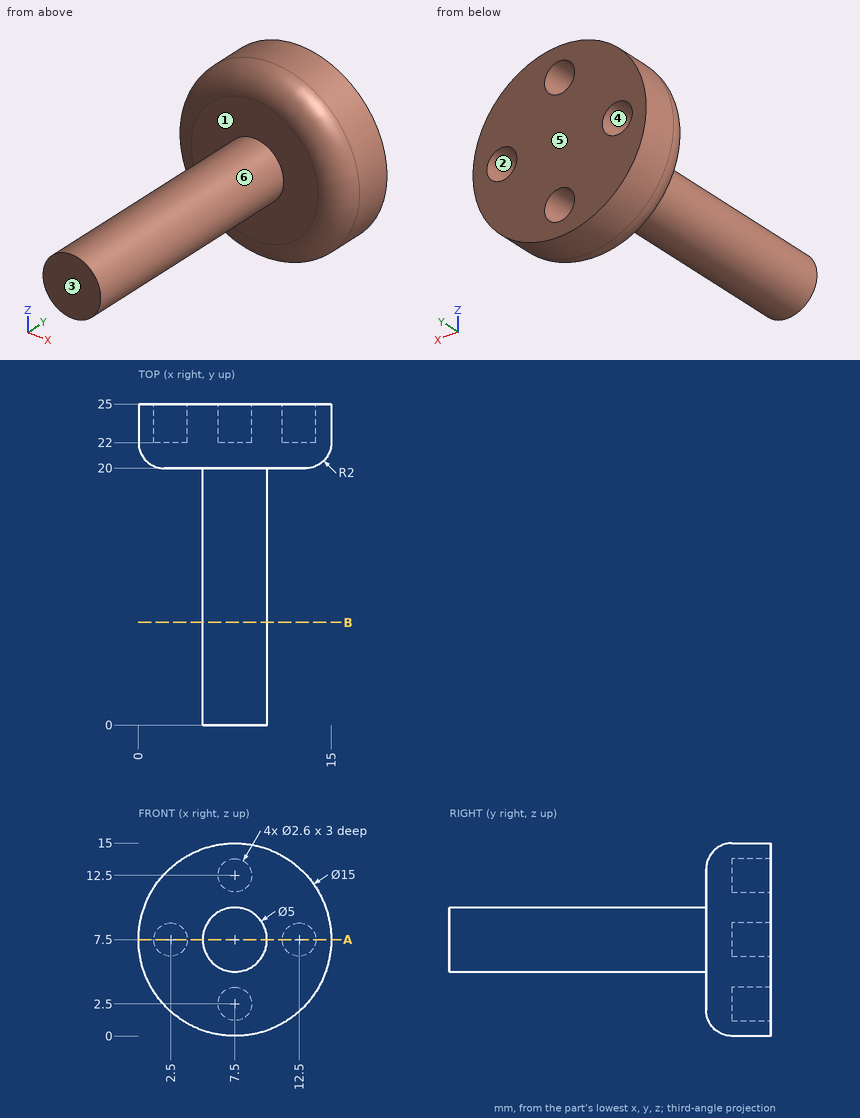
Input: dimensioned drawing with shaded views. Units: mm. Origin: part minimum x, y, z. A direction names the side the tool comes from. Round coordinates to 2 decimals unless told otherwise and drop trailing zeros. Order: outer loops, then holes, each group sorted by start corner. A loop starts at its lowest first (then second) coordinate and runs counter-clockwise, first axis right, second up.
1. Cut plane B-B, the plane y = 8. Output: boundary loops of the cut face in (x, z).
The answers:
outline: circle Ø5 at (7.5, 7.5)
2. Set-up query: the marked faces 1, 2 and 3. Return all of +Z, -Z, +X, -X, +Y, -Y with unobstructed straight access to the full face (end or side cutting, diameter ignored); none if empty.
The answers:
face 1: -Y
face 2: +Y
face 3: +Z, -Z, +X, -X, -Y
3. Mould query, pull axis Z, two halves, no side actions, for the marked faces 4, 5 and 6. Classes: released by +Z, released by -Z, zero draft, split by the parting line, or undercut.
The answers:
face 4: undercut
face 5: zero draft
face 6: split by the parting line
4. Pin query (flat end, axial travel): P1, Ø2, axis at x = 7, z = 2, coming from the +Y side; P2, Ø0.8, axis at x = 13, z = 8, coming from the +Y side; P3, Ø5, axis at y = 12, z = 2, coming from the -X side; P4, Ø3, axis at x = 7.5, z = 2.5, coming from the -Y side. Return the tip coordinate at first contact, or that it passes through.
The answers:
P1: stops at y = 25
P2: stops at y = 22
P3: passes through
P4: stops at y = 20
5. Material intervals for line 1 (X direction, y = 23, z = 7.5); line 2 (Y direction, x = 6.5, z = 3); line 3 (Y direction, x = 3.5, z = 6), sorted ascending.
The answers:
line 1: x = 0 to 1.2, 3.8 to 11.2, 13.8 to 15
line 2: y = 20 to 22
line 3: y = 20 to 25
6. Cut plane A-A, the plane z = 7.5. Output: boundary loops of the cut face in (x, y).
The answers:
outline: (0, 22) arc R2 ccw to (2, 20) - (5, 20) - (5, 0) - (10, 0) - (10, 20) - (13, 20) arc R2 ccw to (15, 22) - (15, 25) - (13.8, 25) - (13.8, 22) - (11.2, 22) - (11.2, 25) - (3.8, 25) - (3.8, 22) - (1.2, 22) - (1.2, 25) - (0, 25) - close
